Autodesk Inventor part; units mm, degrees
ref_plane "YZ Plane" through (0, 0, 0) normal (1, 0, 0) x (0, 1, 0)
ref_plane "XZ Plane" through (0, 0, 0) normal (0, 1, 0) x (-1, 0, 0)
ref_plane "XY Plane" through (0, 0, 0) normal (0, 0, 1) x (1, 0, 0)
sketch "Skizze1" plane through (0, 0, 0) normal (0, 1, 0) x (-1, 0, 0)
  line L0 (15.25, -16.5) -> (-15.25, -16.5)
  line L1 (15.25, 16.5) -> (-15.25, 16.5)
  arc A0 (-18.421, -10.0619) -> (-18.421, 10.0619) centre (-31.5074, 0) ccw
  arc A1 (18.421, 10.0619) -> (18.421, -10.0619) centre (31.5074, 0) ccw
  arc A2 (15.25, -16.5) -> (18.421, -10.0619) centre (15.25, -12.5) ccw
  arc A3 (18.421, 10.0619) -> (15.25, 16.5) centre (15.25, 12.5) ccw
  arc A4 (-15.25, 16.5) -> (-18.421, 10.0619) centre (-15.25, 12.5) ccw
  arc A5 (-18.421, -10.0619) -> (-15.25, -16.5) centre (-15.25, -12.5) ccw
  circle A6 centre (15, -12) radius 2.15
  circle A7 centre (-15, -12) radius 2.15
  circle A8 centre (-15, 12) radius 2.15
  circle A9 centre (15, 12) radius 2.15
  line L2 (15, 12) -> (15, -12) construction
  line L3 (15, -12) -> (-15, -12) construction
  line L4 (-15, -12) -> (-15, 12) construction
  line L5 (-15, 12) -> (15, 12) construction
  line L6 (0, -24.4811) -> (0, 24.4811)
  line L7 (44.8, 0) -> (-44.8, 0)
  line L8 (15, 0) -> (-15, 0) construction
  point P0 (0, 0)
  point P1 (32, -16.5)
  point P2 (-32, -16.5)
  point P3 (32, 16.5)
  point P4 (-32, 16.5)
  dimension "d0" = 4
  dimension "d1" = 30
  dimension "d2" = 24
  dimension "d3" = 33
  dimension "d4" = 4.3
  dimension "d5" = 38.5
extrude "Extrusion1" add sketch "Skizze1" along normal blind 1.2
sketch "Skizze2" plane through (0, 0, 0) normal (1, 0, 0) x (0, 1, 0)
  line L0 (0, 10.0619) -> (0, -10.0619)
  line L1 (0, 12) -> (-3, 12)
  line L2 (-3, 12) -> (-3, -12)
  line L3 (-3, -12) -> (0, -12)
  line L4 (-1.683, 0) -> (1.6805, 0)
  circle A0 centre (-23.6, -16) radius 16
  line L5 (1.2, 10.0619) -> (1.2, -10.0619)
  line L6 (0, -16.5) -> (1.2, -16.5)
  circle A1 centre (-23.6, -16) radius 5
  line L7 (-3, -12) -> (-3, -20)
  line L8 (-3, -20) -> (-23.3561, -20.994)
  line L9 (-3, 4) -> (-26.405, -11.8609)
  line L10 (0, 0) -> (-3, 0)
  line L11 (0, 10.0619) -> (0, -10.0619)
  line L12 (0, 0) -> (0, -12)
  dimension "d8" = 3
  dimension "d9" = 32
  dimension "d10" = 40.8
  dimension "d12" = 0
  dimension "d13" = 10
  dimension "d14" = 8
  dimension "d16" = 8
  dimension "d18" = 24
revolve "Umdrehung1" add sketch "Skizze2" angle 360 about axis through (0, 0, 0) along (0, -1, 0) contours L0 L12 L3 L2 L10 L4
extrude "Extrusion2" add sketch "Skizze2" along normal mid plane 13 contours L9 A1 L8 A0 | A0 L8 A1 L9
extrude "Extrusion3" add sketch "Skizze2" along normal mid plane 18 contours A1
sketch "Skizze3" plane through (-9, -23.6, -16) normal (-1, 0, 0) x (0, 0, 1)
  line L0 (-4, 20.6) -> (-4.994, 0.2439)
  line L1 (4, 20.6) -> (-4, 20.6)
  line L2 (20, 20.6) -> (4.1391, -2.805)
  circle A0 centre (0, 0) radius 5
  line L3 (-4, 20.6) -> (20, 20.6)
  line L4 (4, 20.6) -> (28, 20.6)
  line L5 (20, 20.6) -> (4.1391, -2.805)
  circle A1 centre (0, 0) radius 5
  arc A2 (4.1391, -2.805) -> (-4.994, 0.2439) centre (0, 0) ccw
  line L6 (-4.994, 0.2439) -> (-4, 20.6)
  point P0 (16, 23.6)
extrude "Extrusion4" add sketch "Skizze3" against normal blind 1.2 contours L1 L3 L2 A0 L0
mirror "Spiegeln1" about plane through (0, 0, 0) normal (1, 0, 0) of "Extrusion4"
sketch "Skizze4" plane through (7.8, -3, -9.1192) normal (-1, 0, 0) x (0, 0, 1)
  line L0 (-10.8808, 0) -> (-11.8748, -20.3561)
  line L1 (-10.9394, -1.2) -> (0, -1.2)
  line L2 (0, 0) -> (1.182, 0)
  line L3 (0, -1.2) -> (0, 0)
  line L4 (1.182, 0) -> (-10.8808, 0)
  point P0 (9.1192, 3)
  dimension "d27" = 1.2
extrude "Extrusion5" add sketch "Skizze4" along normal up to surface (15.6 mm away)
properties part number "Castor_Wheel" material "Stahl, unlegiert"
Here's how the part is built. I have some questions about the finished solid (model axes, mm). A direction names the side the tool comes from. Give positions to 0.01 mm unless a question says otherwise; leave off trailing zeros. Write each loop counter-clockwise with the first axis right and the second up, starting at its lowest first coordinate (ties: lowest second). Pieces come first, ordered by that corner, then holes. Notation, with made-up numbers: (-8, 38) -> (11, 38) arc R20 ccw to (11, 56) -> close; hole circle Ø9 at (81, -27.5). An arc over 180 degrees is marked (long way). Use one line per item in the form item = value.
1) Suppose I cut it at B-B (x = -16). Please give me the cut outline in (y, z), and give its area (3 significant figures).
Verdict:
outline = (0, -16.43) -> (1.2, -16.43) -> (1.2, -13.9) -> (0, -13.9) -> close; (0, -10.1) -> (1.2, -10.1) -> (1.2, -5.66) -> (0, -5.66) -> close; (0, 5.66) -> (1.2, 5.66) -> (1.2, 10.1) -> (0, 10.1) -> close; (0, 13.9) -> (1.2, 13.9) -> (1.2, 16.43) -> (0, 16.43) -> close
area = 16.7 mm2
2) If I drill on L1, parallel to X at y = -20.5, z = -8; L2, parallel to Y at x = 13, z = 14.5; L3, parallel to X at y = -33, z = -17.5, over which ranges is the centre line in solid material (lowest first)? Write a range as [from, to].
Verdict:
L1 = [-9, -7.8], [-6.5, 6.5], [7.8, 9]
L2 = [0, 1.2]
L3 = [-6.5, 6.5]
3) Suppose I cut it at A-A (x = 0). Please give me the cut outline in (y, z), and give its area (3 significant figures).
Verdict:
outline = circle Ø32 at (-23.6, -16); (-4.2, -20.06) -> (-3, -20) -> (-3, -12) -> (0, -12) -> (0, -16.5) -> (1.2, -16.5) -> (1.2, 16.5) -> (0, 16.5) -> (0, 12) -> (-3, 12) -> (-3, -9.12) -> (-4.2, -9.12) -> close
area = 929 mm2
4) We'd pull the mould along X, two halves only. Please class faces 4 (the face through (12.95, 0.59, 11.35)), 5 (the face through (-18.81, 0.59, 14.32)), 6 (the face through (0, 1, -16.5)): +X half, -X half, draft (parallel to the pull), parting line (faces both ways), or undercut.
Verdict:
face_4 = undercut
face_5 = -X half
face_6 = draft
5) Suppose I cut it at D-D (z = -19). Please give me the cut outline in (x, y).
Verdict:
outline = (-9, -27.6) -> (-6.5, -27.6) -> (-6.5, -39.32) -> (6.5, -39.32) -> (6.5, -27.6) -> (9, -27.6) -> (9, -3) -> (-9, -3) -> close; hole (-7.8, -19.6) -> (-6.5, -19.6) -> (-6.5, -7.88) -> (6.5, -7.88) -> (6.5, -19.6) -> (7.8, -19.6) -> (7.8, -4.2) -> (-7.8, -4.2) -> close
6) On a 3-axis mill with a long thin cutter (end or side, diameter ignored), from which of +Z, -Z, +X, -X, +Y, -Y can I reach the whole of each face in a straight line? I mean faces 1 (the face through (0, -4, -9.119)), 2 (the face through (-7.49, -27.285, -19.379)), 3 (the face through (0, -4.2, -15)). Say none if no direction works.
Verdict:
face_1 = +Z
face_2 = none
face_3 = +Z, -Z
7) Suppose I cut it at C-C (y = -20). Please give me the cut outline in (x, z).
Verdict:
outline = (-9, -20.83) -> (-7.8, -20.83) -> (-7.8, -19.47) -> (-6.5, -19.47) -> (-6.5, -31.59) -> (6.5, -31.59) -> (6.5, -19.47) -> (7.8, -19.47) -> (7.8, -20.83) -> (9, -20.83) -> (9, -7.52) -> (7.8, -7.52) -> (7.8, -12.53) -> (6.5, -12.53) -> (6.5, -0.41) -> (-6.5, -0.41) -> (-6.5, -12.53) -> (-7.8, -12.53) -> (-7.8, -7.52) -> (-9, -7.52) -> close
8) I'm going to push flat-ended pins straight in: pin 1 (7 mm diameter, centred on y = -12, z = -13, fed in from +X); pin 2 (2.5 mm diameter, centred on x = -15, z = 12, fed in from -Y); pin 3 (10 mm diameter, centred on y = -4.5, z = -15, fed in from -X); pin 4 (12 mm diameter, centred on x = 0, z = 8.5, fed in from -Y). Where does each tip first touch, or does it pass through?
Verdict:
pin_1 = 9
pin_2 = through
pin_3 = -19.24
pin_4 = -3
